Source: three-view drawing plus pictorial views. Frame: mm from the lowest corner of the part. A direction names the side the tool comes from. Round coordinates to 2 decimals unless told otherwise and drop trailing zeros. Order: outer loops, then holes, each group sorted by start corner. A loop starts at its lowest first (then second) coordinate and runs counter-clockwise, first axis right, second up. Notation, with made-up numbers: M -12.5,42.25 L 10.5,42.25 A20 ccw 10.5,50.25 Z; hole C 54.25,9 d5. An arc over 180 degrees is marked long. Return JSON: item names as keys, results as strings. Group by question number.
Q1. Access query for the marked faces 1 and 2. Directions: +Z, -Z, +X, -X, +Y, -Y. A direction counts if a zero-diameter tool reaches every point of the face in a straight line with its end or side. Return the directions, or none.
Q2. Ray query, probe 1 along Z at (x, y) = (62.5, 8.5); probe 2 along Z at (x, y) = (90, 24) (1 decimal); probe 3 along Z at (x, y) = (48.5, 12.5). Return the intervals inside material, ascending.
Q3. Cut plane C-C on x = 38. Output: boundary loops of the cut face in (y, z), and give its area (3 significant figures).
Q4. Cut plane A-A on x = 10.5. Output: boundary loops of the cut face in (y, z).
Q5. Contact query for flat-ended pins moving along their axis: pin 1 (5 mm diameter, centred on x = 36.73, z = 47.23, fed in from +Y); pin 2 (1.5 mm diameter, centred on x = 27, y = 51.5, fed in from +Z); pin 3 (9 mm diameter, centred on x = 62.73, z = 73.23, fed in from +Y). Output: stop coordinate, or through.
Q6. Cut plane B-B on y = 14. Count the separate pieces of the cut face and the enclosed holes in it, and give its area (3 significant figures).
Q7. Cut plane D-D on z = 27. Output: boundary loops of the cut face in (x, y).
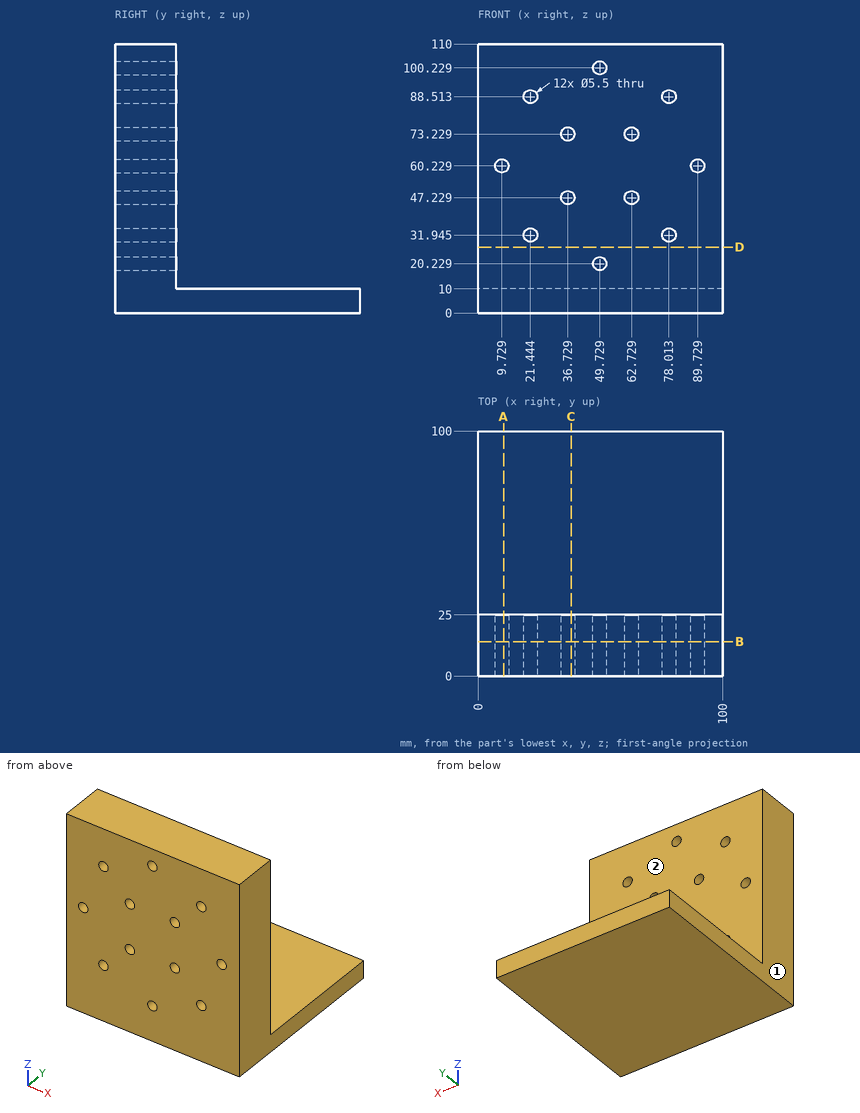
Result sheet:
{
 "1": {"face 1": "+Z, -Z, -X, +Y, -Y", "face 2": "+Z, +X, -X, +Y"},
 "2": {"probe 1": "z = 0 to 44.49, 49.97 to 70.49, 75.97 to 110", "probe 2": "z = 0 to 57.5, 63 to 110", "probe 3": "z = 0 to 17.77, 22.69 to 97.77, 102.69 to 110"},
 "3": {"outline": "M 0,0 L 100,0 L 100,10 L 25,10 L 25,44.79 L 0,44.79 Z; M 0,49.67 L 25,49.67 L 25,70.79 L 0,70.79 Z; M 0,75.67 L 25,75.67 L 25,110 L 0,110 Z", "area": "3,260 mm²"},
 "4": {"outline": "M 0,0 L 100,0 L 100,10 L 25,10 L 25,57.59 L 0,57.59 Z; M 0,62.87 L 25,62.87 L 25,110 L 0,110 Z"},
 "5": {"pin 1": "passes through", "pin 2": "stops at z = 10", "pin 3": "stops at y = 25"},
 "6": {"separate pieces": "1", "enclosed holes": "12", "area": "10,700 mm²"},
 "7": {"outline": "M 0,0 L 100,0 L 100,25 L 0,25 Z"}
}
